Could you check a few things on this model? Use its own coordinates, in mm. Round coordinates to 2 decimals unless told otherwise and drop trailing zeros. Loops run counter-clockwise (first coordinate to the right, second up) from the corner with the lowest first, then second, coordinate; pieces in that order, holes last. Notation, with made-up numbers: M 61.5,65.25 L 69.5,65.25 A6 cw 69.5,69.25 Z; hole C 71,-4 d3. An arc over 180 degrees is marked long. Answer in a Markdown table with one row per item.
```python
from build123d import *

# Parameters (mm, degrees)
SKETCH1_W           = 173.4
SKETCH1_H           = 101.6
BOSS_EXTRUDE1_DEPTH = 3
SKETCH2_W           = 2.92
SKETCH2_H           = 50.64
CUT_EXTRUDE1_DEPTH  = 3
LPATTERN1_COUNT     = 6
LPATTERN1_PITCH     = 34.096


with BuildPart() as part:
    # Sketch1 → Boss-Extrude1 (new body)
    with BuildSketch(Plane(origin=(0, 0, 0), x_dir=(1, 0, 0), z_dir=(0, 1, 0))):
        with Locations((86.7, 50.8)):
            Rectangle(SKETCH1_W, SKETCH1_H)
    extrude(amount=BOSS_EXTRUDE1_DEPTH)

    # Sketch2 → Cut-Extrude1 (cut)
    with BuildSketch(Plane(origin=(0, 3, 0), x_dir=(1, 0, 0), z_dir=(0, 1, 0))):
        with Locations((1.46, 50.8)):
            Rectangle(SKETCH2_W, SKETCH2_H)
    cut_extrude1 = extrude(amount=-CUT_EXTRUDE1_DEPTH, mode=Mode.SUBTRACT)

    # LPattern1: Cut-Extrude1 ×6
    with Locations(*[(i * LPATTERN1_PITCH, 0, 0) for i in range(1, LPATTERN1_COUNT)]):
        add(cut_extrude1, mode=Mode.SUBTRACT)


solid = part.part
```
1) Will these pins go through, and if not, where does the flat tip stop? P1, Ø1.5, axis at y = 1.5, z = -56.5, coming from the -X side; P2, Ø1.5, axis at y = 1, z = -43.5, coming from the +X side.
Computed:
| item | result |
|---|---|
| P1 | stops at x = 2.92 |
| P2 | stops at x = 170.48 |
2) I need wall thicknesses on line 1 (X direction, y = 1.4, z = -34); line 2 (Z direction, x = 68.5, y = 0.3). Which ranges of each line are inside material? Lowest first, please.
Computed:
| item | result |
|---|---|
| line 1 | x = 2.92 to 34.1, 37.02 to 68.19, 71.11 to 102.29, 105.21 to 136.38, 139.3 to 170.48 |
| line 2 | z = -101.6 to -76.12, -25.48 to 0 |
3) I want a section at B-B, the plane y = 2.45. Please give me the cut outline in (x, z), plus the area to 3 significant figures.
Computed:
| item | result |
|---|---|
| outline | M 0,-101.6 L 173.4,-101.6 L 173.4,-76.12 L 170.48,-76.12 L 170.48,-25.48 L 173.4,-25.48 L 173.4,0 L 0,0 L 0,-25.48 L 2.92,-25.48 L 2.92,-76.12 L 0,-76.12 Z; hole M 34.1,-76.12 L 37.02,-76.12 L 37.02,-25.48 L 34.1,-25.48 Z; hole M 68.19,-76.12 L 71.11,-76.12 L 71.11,-25.48 L 68.19,-25.48 Z; hole M 102.29,-76.12 L 105.21,-76.12 L 105.21,-25.48 L 102.29,-25.48 Z; hole M 136.38,-76.12 L 139.3,-76.12 L 139.3,-25.48 L 136.38,-25.48 Z |
| area | 16,700 mm² |
4) I want a section at A-A, the plane z = -40.5. Please give me the cut outline in (x, y).
Computed:
| item | result |
|---|---|
| outline | M 2.92,0 L 34.1,0 L 34.1,3 L 2.92,3 Z; M 37.02,0 L 68.19,0 L 68.19,3 L 37.02,3 Z; M 71.11,0 L 102.29,0 L 102.29,3 L 71.11,3 Z; M 105.21,0 L 136.38,0 L 136.38,3 L 105.21,3 Z; M 139.3,0 L 170.48,0 L 170.48,3 L 139.3,3 Z |
